```python
from build123d import *

# Parameters (mm, degrees)
SKETCH_1_R      = 10
EXTRUDE_1_DEPTH = 15


with BuildPart() as part:
    # Эскиз1 → Бобышка-Вытянуть1 (new body, symmetric)
    with BuildSketch(Plane.XY):
        with BuildLine():
            Line((0, 20), (-290, 20))
            ThreePointArc((-290, 20), (-310, 0), (-290, -20))
            Line((-290, -20), (0, -20))
            ThreePointArc((0, -20), (20, 0), (0, 20))
        make_face()
        with Locations((-290, 0)):
            Circle(SKETCH_1_R, mode=Mode.SUBTRACT)
        Circle(SKETCH_1_R, mode=Mode.SUBTRACT)
    extrude(amount=EXTRUDE_1_DEPTH, both=True)


solid = part.part
```
CAD build for the part. Positions are in the model's coordinates, mm. Round coordinates to 2 decimals unless told otherwise and drop trailing zeros. Loops run counter-clockwise (first coordinate to the right, second up) from the corner with the lowest first, then second, coordinate; pieces in that order, holes last. Notation, with made-up numbers: M 27.5,-33.5 L 43.5,-33.5 A20 ccw 43.5,-29.5 Z; hole C 43,-26 d6. An arc over 180 degrees is marked long. Use a Markdown table: item, result. Add a question column.
(1) Pull direction X, two halves, no side cores. Call faces 1 (the face through (20, 0, 0)), 2 (the face through (-310, 0, 0)), 3 (the face through (-300, 0, 0)): +X half, -X half, draft (parallel to the pull), parting line (faces both ways), or undercut.
(2) Cut at C-C (y = 14). Give the cut face in (x, z).
(3) Cut at A-A (y = -5). Give the cut face in (x, z), and give its area (3 significant figures).
(4) Cut at B-B (z = 3). Give the cut face in (x, y), and give its area (3 significant figures).
(5) Flat gauge pins, fed straight in: pin 1 (2 mm diameter, centred on y = 6.5, z = 8.5, fed in from +X); pin 2 (12 mm diameter, centred on x = 0, y = 0, fed in from -Z); pin 3 (1.5 mm diameter, centred on y = -10.5, z = -7.5, fed in from -X); pin 4 (5 mm diameter, centred on y = -6.5, z = 8, fed in from +X). Where does each tip first touch, or does it go through?
(6) Drill centre lines: line 1 (X direction, y = -0.5, z = 4.5); line 2 (X direction, y = -1, z = -7); line 3 (Y direction, x = -290, z = -0.5). Where is each one in solid material? Low to high.
Geometry says:
| question | item | result |
|---|---|---|
| 1 | face 1 | +X half |
| 1 | face 2 | -X half |
| 1 | face 3 | undercut |
| 2 | outline | M -304.28,-15 L 14.28,-15 L 14.28,15 L -304.28,15 Z |
| 3 | outline | M -309.36,-15 L -298.66,-15 L -298.66,15 L -309.36,15 Z; M -281.34,-15 L -8.66,-15 L -8.66,15 L -281.34,15 Z; M 8.66,-15 L 19.36,-15 L 19.36,15 L 8.66,15 Z |
| 3 | area | 8,820 mm² |
| 4 | outline | M -290,-20 L 0,-20 A20 ccw 0,20 L -290,20 A20 ccw Z; hole C -290,0 d20; hole C 0,0 d20 |
| 4 | area | 12,200 mm² |
| 5 | pin 1 | stops at x = 19.23 |
| 5 | pin 2 | passes through |
| 5 | pin 3 | stops at x = -307.46 |
| 5 | pin 4 | stops at x = 19.6 |
| 6 | line 1 | x = -309.99 to -299.99, -280.01 to -9.99, 9.99 to 19.99 |
| 6 | line 2 | x = -309.97 to -299.95, -280.05 to -9.95, 9.95 to 19.97 |
| 6 | line 3 | y = -20 to -10, 10 to 20 |
